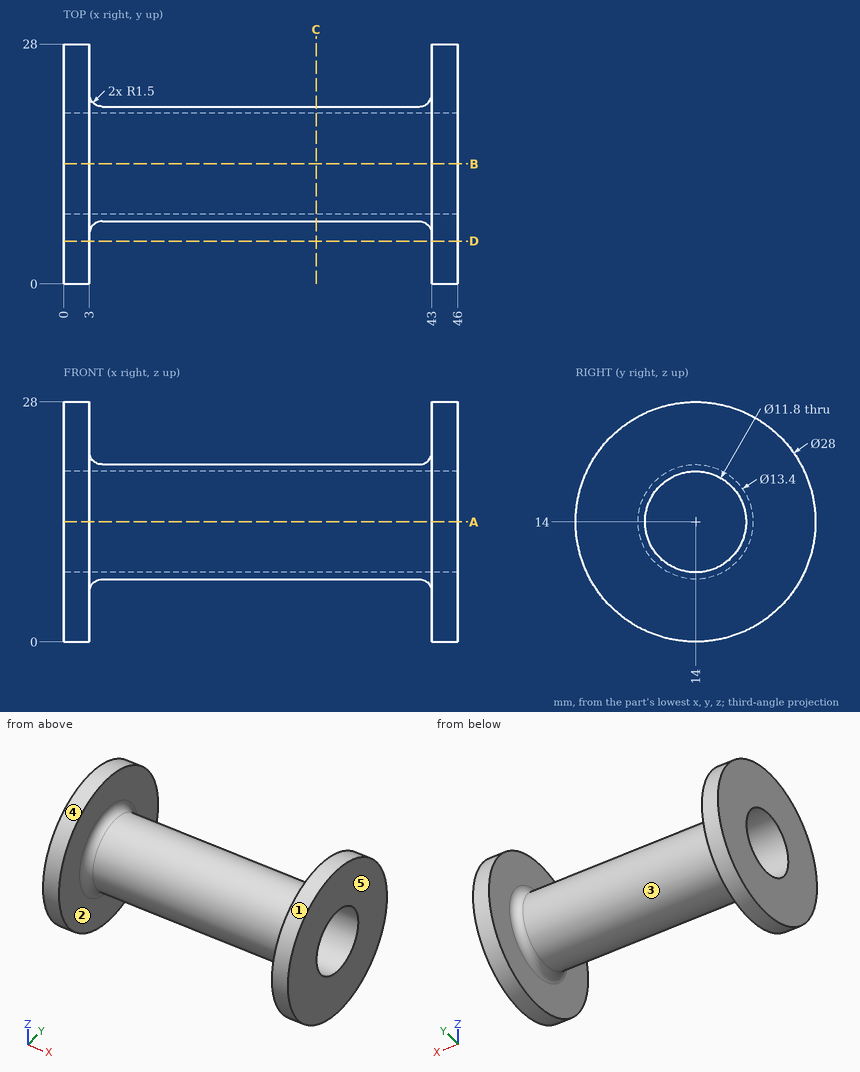
Verification items for this drawing (mm, ordinates from the low corner). A direction names the side the tool comes from. Give positions to 0.01 mm unless a question says otherwise; leave off trailing zeros. Write each loop counter-clockwise with the first axis right and the second up, starting at its lowest first coordinate (ties: lowest second). Pieces come first, ordered by that corner, then holes. Notation, with made-up numbers: (74.25, -37) -> (126.25, -37) arc R10 ccw to (126.25, -21) -> close; hole circle Ø3 at (12.5, 0.5). An arc over 180 degrees is marked (long way). Use CSV: the item, a comma, the result in double quotes.
(1) Release check for a two-part mould opening along X. For the marked faces 3, 4 and 5 record: +X half, -X half, draft (parallel to the pull), parting line (faces both ways), or undercut.
Derived:
face 3,"undercut"
face 4,"draft"
face 5,"+X half"
(2) Sectioned sample at C-C (x = 29.5). Record the cut outline in (y, z), plus the area to 3 significant figures.
Derived:
outline,"circle Ø13.4 at (14, 14); hole circle Ø11.8 at (14, 14)"
area,"31.7 mm^2"
(3) Go/stop test with flat-tipped pins: pin 1 (6 mm diameter, centred on x = 32.5, y = 11.5, fed in from -Z); pin 2 (12 mm diameter, centred on x = 20, y = 6.5, fed in from -Z); pin 3 (1.5 mm diameter, centred on x = 24.5, z = 10.5, fed in from -Y); pin 4 (8.5 mm diameter, centred on y = 13, z = 13, fed in from -X). Record where each tip stops, or that it passes through.
Derived:
pin 1,"stops at z = 7.3"
pin 2,"stops at z = 7.47"
pin 3,"stops at y = 7.89"
pin 4,"passes through"
(4) Set-up check for the marked faces 1 and 2: record each of +Z, -Z, +X, -X, +Y, -Y from which the full face is reachable in a straight line by a thin tool's end or side.
Derived:
face 1,"+X, -X"
face 2,"none"
(5) Sectioned sample at A-A (z = 14). Record the cut outline in (x, y).
Derived:
outline,"(0, 0) -> (3, 0) -> (3, 5.8) arc R1.5 cw to (4.5, 7.3) -> (41.5, 7.3) arc R1.5 cw to (43, 5.8) -> (43, 0) -> (46, 0) -> (46, 8.1) -> (0, 8.1) -> close; (0, 19.9) -> (46, 19.9) -> (46, 28) -> (43, 28) -> (43, 22.2) arc R1.5 cw to (41.5, 20.7) -> (4.5, 20.7) arc R1.5 cw to (3, 22.2) -> (3, 28) -> (0, 28) -> close"
(6) Material ranges on L1, parallel to Y at x = 26.5, z = 14; L2, parallel to X at y = 12, z = 22.25, recorded low to high.
Derived:
L1,"y = 7.3 to 8.1, 19.9 to 20.7"
L2,"x = 0 to 3, 43 to 46"
(7) Sectioned sample at D-D (y = 5). Record the cut outline in (x, z), plus the area to 3 significant figures.
Derived:
outline,"(0, 3.28) -> (3, 3.28) -> (3, 24.72) -> (0, 24.72) -> close; (43, 3.28) -> (46, 3.28) -> (46, 24.72) -> (43, 24.72) -> close"
area,"129 mm^2"
